Source: CAD feature listing. Evaluate the final solid. Frame: model axes, mm. A direction names the side the tool comes from. Round coordinates to 2 decimals unless told otherwise and drop trailing zeros. Write each loop counter-clockwise with the first axis right and the second up, starting at its lowest first coordinate (ties: lowest second). Pieces come first, ordered by that corner, then holes. Notation, with made-up numbers: M 29,-38 L 68,-38 A9 ccw 68,-32 Z; hole C 21,84.25 d9. An arc over 180 degrees is marked long. Answer in a Markdown table with one row per item.
from build123d import *

# Parameters (mm, degrees)
SKETCH1_W           = 60
SKETCH1_H           = 70
BOSS_EXTRUDE3_DEPTH = 60
SKETCH2_W           = 50
SKETCH2_H           = 50
CUT_EXTRUDE1_DEPTH  = 5
SKETCH3_W           = 5
SKETCH3_H           = 10
CUT_EXTRUDE3_DEPTH  = 111
SKETCH6_W           = 5
SKETCH6_H           = 10
CUT_EXTRUDE4_DEPTH  = 111
CUT_EXTRUDE5_DEPTH  = 5
CUT_EXTRUDE7_DEPTH  = 5
SKETCH9_W           = 40
SKETCH9_H           = 40
CUT_EXTRUDE8_DEPTH  = 60
SKETCH10_R          = 5
CUT_EXTRUDE9_DEPTH  = 111


with BuildPart() as part:
    # Sketch1 → Boss-Extrude3 (new body)
    with BuildSketch(Plane.XY):
        with Locations((30, 35)):
            Rectangle(SKETCH1_W, SKETCH1_H)
    extrude(amount=BOSS_EXTRUDE3_DEPTH)

    # Sketch2 → Cut-Extrude1 (cut)
    with BuildSketch(Plane(origin=(0, 70, 0), x_dir=(1, 0, 0), z_dir=(0, 1, 0))):
        with Locations((30, -30)):
            Rectangle(SKETCH2_W, SKETCH2_H)
    extrude(amount=-CUT_EXTRUDE1_DEPTH, mode=Mode.SUBTRACT)

    # Sketch3 → Cut-Extrude3 (cut, through all)
    with BuildSketch(Plane.XY.offset(60)):
        with Locations((2.5, 15)):
            Rectangle(SKETCH3_W, SKETCH3_H)
        with Locations((57.5, 15)):
            Rectangle(SKETCH3_W, SKETCH3_H)
    extrude(amount=-CUT_EXTRUDE3_DEPTH, mode=Mode.SUBTRACT)

    # Sketch6 → Cut-Extrude4 (cut, through all)
    with BuildSketch(Plane(origin=(60, 0, 0), x_dir=(0, 0, -1), z_dir=(1, 0, 0))):
        with Locations((-57.5, 15)):
            Rectangle(SKETCH6_W, SKETCH6_H)
        with Locations((-2.5, 15)):
            Rectangle(SKETCH6_W, SKETCH6_H)
    extrude(amount=-CUT_EXTRUDE4_DEPTH, mode=Mode.SUBTRACT)

    # Sketch7 → Cut-Extrude5 (cut)
    with BuildSketch(Plane(origin=(60, 0, 0), x_dir=(0, 0, -1), z_dir=(1, 0, 0))):
        Polygon((-36, 40), (-24, 40), (-24, 43), (-20, 43), (-20, 40), (-20, 35), (-40, 35), (-40, 40), (-40, 43), (-36, 43), align=None)
    extrude(amount=-CUT_EXTRUDE5_DEPTH, mode=Mode.SUBTRACT)

    # Sketch8 → Cut-Extrude7 (cut)
    with BuildSketch(Plane(origin=(60, 0, 0), x_dir=(0, 0, -1), z_dir=(1, 0, 0))):
        with BuildLine():
            Line((-45, 55), (-45, 62.5))
            ThreePointArc((-45, 62.5), (-48.408526169, 48.319285266), (-38.927629067, 59.401853162))
            Line((-38.927629067, 59.401853162), (-45, 55))
        make_face()
        with BuildLine():
            Line((-15, 55), (-8.927629067, 59.401853162))
            ThreePointArc((-8.927629067, 59.401853162), (-18.408526169, 48.319285266), (-15, 62.5))
            Line((-15, 62.5), (-15, 55))
        make_face()
    extrude(amount=-CUT_EXTRUDE7_DEPTH, mode=Mode.SUBTRACT)

    # Sketch9 → Cut-Extrude8 (cut)
    with BuildSketch(Plane(origin=(0, 0, 0), x_dir=(-1, 0, 0), z_dir=(0, -1, 0))):
        with Locations((-30, -30)):
            Rectangle(SKETCH9_W, SKETCH9_H)
    extrude(amount=-CUT_EXTRUDE8_DEPTH, mode=Mode.SUBTRACT)

    # Sketch10 → Cut-Extrude9 (cut, through all)
    with BuildSketch(Plane.XY.offset(60)):
        with Locations((30, 45)):
            Circle(SKETCH10_R)
    extrude(amount=-CUT_EXTRUDE9_DEPTH, mode=Mode.SUBTRACT)


solid = part.part
Q1. Section A-A (y = 45). Return loops of the section in (x, z), and give its area (3 significant figures).
Solutions:
| item | result |
|---|---|
| outline | M 0,0 L 25,0 L 25,10 L 10,10 L 10,50 L 25,50 L 25,60 L 0,60 Z; M 35,0 L 60,0 L 60,60 L 35,60 L 35,50 L 50,50 L 50,10 L 35,10 Z |
| area | 1,800 mm2 |
Q2. Section C-C (x = 30). Return loops of the section in (y, z).
Solutions:
| item | result |
|---|---|
| outline | M 0,0 L 10,0 L 10,5 L 20,5 L 20,0 L 40,0 L 40,10 L 0,10 Z; M 0,50 L 40,50 L 40,60 L 20,60 L 20,55 L 10,55 L 10,60 L 0,60 Z; M 50,0 L 70,0 L 70,5 L 65,5 L 65,55 L 70,55 L 70,60 L 50,60 L 50,50 L 60,50 L 60,10 L 50,10 Z |
Q3. Pull-direction query (Y, two-part tool) for faces 1 (the flat face through (58, 40, 30)), 2 (the flat face through (55, 68, 30)), 3 (the flat face through (29.6, 0, 9.6)); classes: pulls with the +Y half, pulls with the -Y half, needs draft (parallel to the pull), parting line crosses it, or undercut.
Solutions:
| item | result |
|---|---|
| face 1 | undercut |
| face 2 | needs draft |
| face 3 | pulls with the -Y half |
Q4. Contact query for flat-ended pins moving along their axis: pin 1 Ø12 at (x, z) = (30, 26) entering from +Y; pin 2 Ø8 at (x, y) = (30, 45) entering from +Z. Output: stop coordinate, or through.
Solutions:
| item | result |
|---|---|
| pin 1 | stops at y = 65 |
| pin 2 | passes through |
Q5. Section D-D (z = 33). Return loops of the section in (x, y), and give its area (4 significant figures).
Solutions:
| item | result |
|---|---|
| outline | M 0,0 L 10,0 L 10,60 L 50,60 L 50,0 L 60,0 L 60,10 L 55,10 L 55,20 L 60,20 L 60,35 L 55,35 L 55,40 L 60,40 L 60,70 L 55,70 L 55,65 L 5,65 L 5,70 L 0,70 L 0,20 L 5,20 L 5,10 L 0,10 Z |
| area | 1,425 mm2 |
Q6. Material intervals for probe 1 along Y at (x, z) = (30, 4.75); probe 2 along Y at (x, z) = (30, 8); probe 3 along Y at (x, z) = (28, 56.5), sorted ascending.
Solutions:
| item | result |
|---|---|
| probe 1 | y = 0 to 10, 20 to 40, 50 to 70 |
| probe 2 | y = 0 to 40, 50 to 65 |
| probe 3 | y = 0 to 10, 20 to 40.42, 49.58 to 70 |
Q7. Section B-B (z = 6). Return loops of the section in (x, y), and give its area (3 significant figures).
Solutions:
| item | result |
|---|---|
| outline | M 0,0 L 60,0 L 60,10 L 55,10 L 55,20 L 60,20 L 60,70 L 55,70 L 55,65 L 5,65 L 5,70 L 0,70 L 0,20 L 5,20 L 5,10 L 0,10 Z; hole C 30,45 d10 |
| area | 3,770 mm2 |
Q8. Access query for faces 4 (the flat face through (58, 59, 15)), 5 (the flat face through (30, 15, 55)), 6 (the flat face through (56, 20, 30)), 7 (the flat face through (30, 60, 30)). Directions: +Z, -Z, +X, -X, +Y, -Y. A direction counts if a zero-diameter tool reaches every point of the face in a straight line with its end or side. Return the directions, or none.
Solutions:
| item | result |
|---|---|
| face 4 | +X |
| face 5 | +Z, +X, -X |
| face 6 | none |
| face 7 | -Y |
